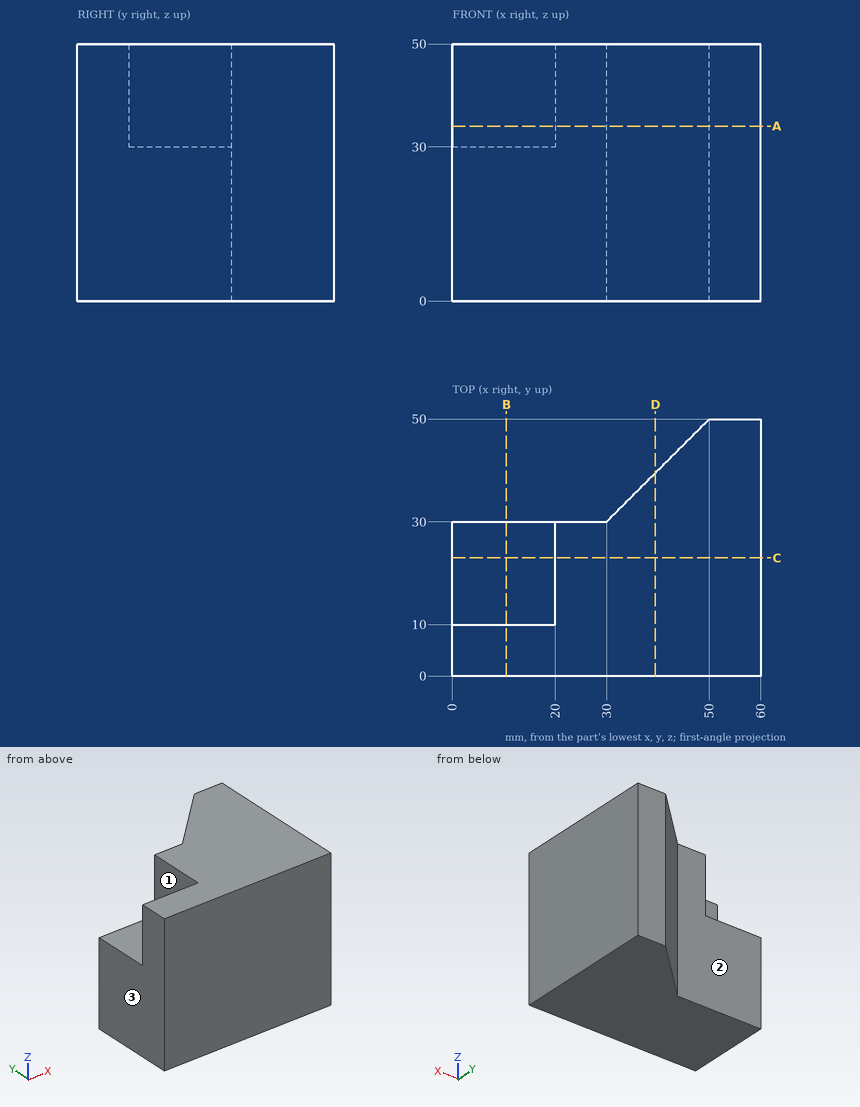
Could you check a few things on this drawing? It's one solid part, dimensions in mm from its lowest x, y, z. A direction names the side the tool comes from. Coordinates: 2 decimals unless noted, no trailing zeros. Order: outer loops, then holes, each group sorted by start corner. A loop starts at its lowest first (then second) coordinate and runs counter-clockwise, first axis right, second up. Notation, with made-up numbers: M -15.75,-35 L 26.25,-35 A13 ccw 26.25,-28 Z; hole C 81.5,22.5 d4. An arc over 180 degrees is marked long. Use one line per item in the form item = value. Start each with the question number.
1. On a 3-axis mill with a long thin cutter (end or side, diameter ignored), from which of +Z, -Z, +X, -X, +Y, -Y can I reach the whole of each face in a straight line? I mean the marked faces 1, 2 and 3. Say none if no direction works.
2. Suppose I cut it at B-B on x = 10.5. Write out the boundary of the cut face in (y, z), then the cut area to 3 significant figures.
3. For pin 1 (4 mm diameter, centred on x = 35, z = 27, fed in from +Y); pin 2 (12 mm diameter, centred on x = 25.5, z = 44.5, fed in from +Y); pin 3 (6 mm diameter, centred on x = 11.5, y = 15.5, fed in from +Z), each with a flat end and sliding along its axis, tell me the tip position at first contact or that it passes through.
4. Suppose I cut it at A-A on z = 34. Write out the boundary of the cut face in (x, y), then the cut area to 3 significant figures.
5. Suppose I cut it at D-D on x = 39.5. Write out the boundary of the cut face in (y, z).
6. Please list where these lines run through material, in increasing order: line 1 (X direction, y = 11, z = 35); line 2 (Y direction, x = 11, z = 3.5).
7. Suppose I cut it at C-C on y = 23. Write out the boundary of the cut face in (x, z), then the cut area to 3 significant figures.
Geometry says:
q1.face_1 = +Z, -X, +Y
q1.face_2 = +Z, -Z, -X, +Y
q1.face_3 = +Z, -Z, -X, +Y, -Y
q2.outline = M 0,0 L 30,0 L 30,30 L 10,30 L 10,50 L 0,50 Z
q2.area = 1,100 mm^2
q3.pin_1 = 37
q3.pin_2 = 31.5
q3.pin_3 = 30
q4.outline = M 0,0 L 60,0 L 60,50 L 50,50 L 30,30 L 20,30 L 20,10 L 0,10 Z
q4.area = 1,800 mm^2
q5.outline = M 0,0 L 39.5,0 L 39.5,50 L 0,50 Z
q6.line_1 = 20 to 60
q6.line_2 = 0 to 30
q7.outline = M 0,0 L 60,0 L 60,50 L 20,50 L 20,30 L 0,30 Z
q7.area = 2,600 mm^2
